The listing builds one solid part. Answer for the finished solid, in the listing's coordinates (mm). A direction names the side the tool comes from. Coordinates: 2 decimals unless noted, no trailing zeros. Order: outer loops, then holes, each group sorted by start corner. A loop starts at its lowest first (then second) coordinate and runs counter-clockwise, first axis right, second up. Notation, with made-up numbers: M -6,-40 L 0,-40 A13 cw 0,-23 Z; hole C 48.25,-4 d3. An arc over 180 degrees is marked long. One line per item, written item: value. Start each with the question number.
Q1. Straight lines are drawn through the part: line 1 along X through (y, z) = (5.25, 0) (3 decimals); line 2 along Y through (x, z) = (9.5, 8.75); line 3 along Z through (x, y) = (-13.5, 3) (3 decimals). For each, find the intervals that lie inside material, in ascending order. Write a range as [from, to].
Q2. The part is cut by section D-D on x = -13.5. Give the vertices of the cut face in (y, z) (3 decimals).
Q3. For faces 4 (the flat face through (0, 0, 0)), 5 (the cylindrical face through (0, 8, 5)), 6 (the flat face through (0, 17.95, 6)), determine the directions among +Z, -Z, +X, -X, +Y, -Y from which every point of the face is accessible in a straight line to the end or side of a thin tool.
Q4. Determine the mould class of faces 1 (the cylindrical face through (14.417, 3.154, 0.12)), 2 (the cylindrical face through (-0.065, 13.615, 5.504)), 3 (the flat face through (-12, 6.7, -1)) for opening direction X: pulls with the +X half, pulls with the -X half, needs draft (parallel to the pull), parting line crosses it, or undercut.
Q5. Each of these flat-tipped pins is pushed along its axis until it touches: pin 1 Ø9 at (x, z) = (-1, -1.5) entering from +Y; pin 2 Ø6 at (x, y) = (0.5, 13.5) entering from -Z; pin 3 Ø0.5 at (y, z) = (-2, 4) entering from -X (3 decimals). Where does it stop, or does it pass through?
Q6. The part is cut by section A-A on z = 0. Give the vertices of the cut face in (x, y) (3 decimals), then the cut area to 3 significant figures.
Q7. The part is cut by section C-C on x = 0. Give the vertices of the cut face in (y, z).
Q8. The part is cut by section B-B on z = -9. Give the vertices of the cut face in (x, y).
```python
from build123d import *

# Parameters (mm, degrees)
BOSS_EXTRUDE1_DEPTH = 6.4
BOSS_EXTRUDE2_START = -6.7
SKETCH4_R           = 2.35
BOSS_EXTRUDE2_DEPTH = 7
SKETCH7_R           = 1.9
SKETCH7_R_2         = 1.25
BOSS_EXTRUDE3_DEPTH = 4.4
SKETCH8_W           = 0.2
SKETCH8_H           = 0.5
BOSS_EXTRUDE4_DEPTH = 3.9


with BuildPart() as part:
    # Sketch1 → Boss-Extrude1 (new body)
    with BuildSketch(Plane(origin=(0, 0, 0), x_dir=(1, 0, 0), z_dir=(0, 1, 0))):
        with BuildLine():
            Line((-4.52879675, 14.3), (4.52879675, 14.3))
            ThreePointArc((4.52879675, 14.3), (0, -15), (-4.52879675, 14.3))
        make_face()
    extrude(amount=BOSS_EXTRUDE1_DEPTH)

    # Sketch3 → Revolve1 (revolve)
    with BuildSketch(Plane.XY.offset(6)):
        Polygon((0, 17.95), (0.5, 17.95), (0.5, 9.4), (1, 9.4), (1, 6.4), (0, 6.4), align=None)
    revolve(axis=Axis((0, 6.4, 6), (0, 1, 0)))

    # Sketch4 → Boss-Extrude2 (add)
    with BuildSketch(Plane(origin=(0, 6.4, 0), x_dir=(1, 0, 0), z_dir=(0, 1, 0)).offset(BOSS_EXTRUDE2_START)):
        with Locations((-13.5, 0)):
            Circle(SKETCH4_R)
    boss_extrude2 = extrude(amount=BOSS_EXTRUDE2_DEPTH)

    # Sketch6 → Ø1.85 (1.85) Diameter Hole1 (revolve, cut)
    with BuildSketch(Plane(origin=(-13.5, -0.3, 0), x_dir=(0, 0, -1), z_dir=(1, 0, 0))):
        Polygon((0, 0), (0, 7), (1.15, 7), (0.925, 6.775), (0.925, 0.225), (1.15, 0), align=None)
    f_1_85_1_85_diameter_hole1 = revolve(axis=Axis((-13.5, -6.65, 0), (0, 1, 0)), mode=Mode.SUBTRACT)

    # Mirror1: Boss-Extrude2, Ø1.85 (1.85) Diameter Hole1 across plane
    add(boss_extrude2.mirror(Plane(origin=(0, 0, 0), x_dir=(0, 0, 1), z_dir=(1, 0, 0))))
    add(f_1_85_1_85_diameter_hole1.mirror(Plane(origin=(0, 0, 0), x_dir=(0, 0, 1), z_dir=(1, 0, 0))), mode=Mode.SUBTRACT)

    # Sketch7 → Boss-Extrude3 (add)
    with BuildSketch(Plane.XZ):
        with Locations((0, 10)):
            Circle(SKETCH7_R)
        with Locations((9, -9)):
            Circle(SKETCH7_R_2)
    extrude(amount=BOSS_EXTRUDE3_DEPTH)

    # Sketch8 → Boss-Extrude4 (add)
    with BuildSketch(Plane(origin=(0, 0, 0), x_dir=(-1, 0, 0), z_dir=(0, -1, 0))):
        with Locations((-11.425, -3.85)):
            Rectangle(SKETCH8_W, SKETCH8_H)
        with Locations((11.425, -3.85)):
            Rectangle(SKETCH8_W, SKETCH8_H)
        with Locations((-11.425, 3.85)):
            Rectangle(SKETCH8_W, SKETCH8_H)
        with Locations((11.425, 3.85)):
            Rectangle(SKETCH8_W, SKETCH8_H)
    extrude(amount=BOSS_EXTRUDE4_DEPTH)


solid = part.part
```
Output:
1. line 1: x = [-15.85, -14.425], [-12.575, 12.575], [14.425, 15.85]
1. line 2: y = [0, 6.4]
1. line 3: z = [-6.538, -0.925], [0.925, 6.538]
2. outline: M -0.3,-2.35 L 0,-2.35 L 0,-6.538 L 6.4,-6.538 L 6.4,-2.35 L 6.7,-2.35 L 6.7,-1.15 L 6.475,-0.925 L -0.075,-0.925 L -0.3,-1.15 Z; M -0.3,1.15 L -0.075,0.925 L 6.475,0.925 L 6.7,1.15 L 6.7,2.35 L 6.4,2.35 L 6.4,6.538 L 0,6.538 L 0,2.35 L -0.3,2.35 Z
3. face 4: -Y
3. face 5: +Y
3. face 6: +Z, -Z, +X, -X, +Y
4. face 1: undercut
4. face 2: parting line crosses it
4. face 3: needs draft
5. pin 1: stops at y = 6.4
5. pin 2: stops at z = 5.5
5. pin 3: stops at x = -11.525
6. outline: M -15.85,-0.3 L -14.65,-0.3 L -14.425,-0.075 L -14.425,6.475 L -14.65,6.7 L -15.85,6.7 Z; M -12.575,-0.075 L -12.35,-0.3 L -11.15,-0.3 L -11.15,0 L 11.15,0 L 11.15,-0.3 L 12.35,-0.3 L 12.575,-0.075 L 12.575,6.475 L 12.35,6.7 L 11.15,6.7 L 11.15,6.4 L -11.15,6.4 L -11.15,6.7 L -12.35,6.7 L -12.575,6.475 Z; M 14.425,-0.075 L 14.65,-0.3 L 15.85,-0.3 L 15.85,6.7 L 14.65,6.7 L 14.425,6.475 Z
6. area: 182 mm^2
7. outline: M -4.4,8.1 L 0,8.1 L 0,-14.3 L 6.4,-14.3 L 6.4,5 L 9.4,5 L 9.4,5.5 L 17.95,5.5 L 17.95,6.5 L 9.4,6.5 L 9.4,7 L 6.4,7 L 6.4,15 L 0,15 L 0,11.9 L -4.4,11.9 Z
8. outline: M -12,0 L 7.75,0 L 7.75,-4.4 L 10.25,-4.4 L 10.25,0 L 12,0 L 12,6.4 L -12,6.4 Z
